Geometry check sheet. Reference: drawing and pictorial views, mm from the part's lowest x, y, z. A direction names the side the tool comes from. Round coordinates to 2 decimals unless told otherwise and drop trailing zeros. Order: outer loops, then holes, each group sorted by start corner. A loop starts at its lowest first (then second) coordinate and runs counter-clockwise, first axis right, second up. Notation, with made-up numbers: M -35.5,82 L 6.5,82 A21 cw 6.5,90 Z; hole C 45.25,28 d8. An arc over 180 degrees is marked long. Answer as a JSON object with one key per item and string values. Group by question number.
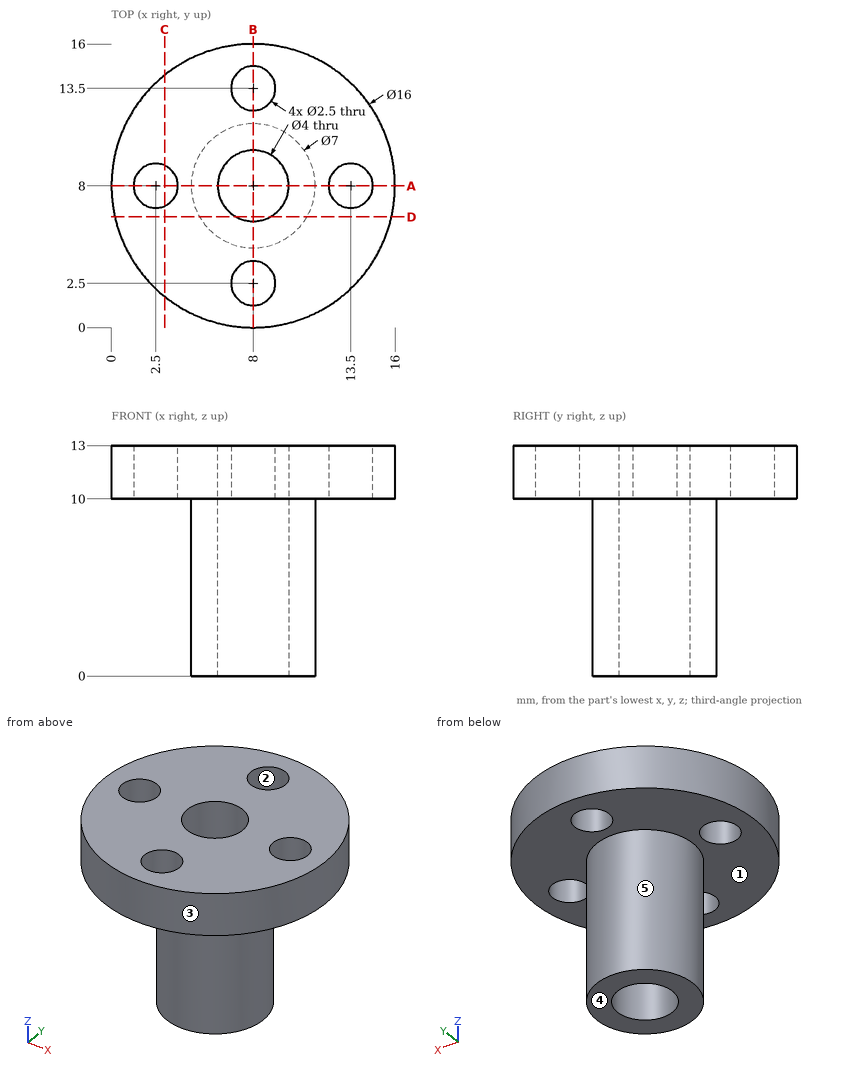
Q1. Tool access check on the marked faces 4 and 5. Record the directions out of +Z, -Z, +X, -X, +Y, -Y that give a thin tool (end or side, any length) a straight path to the whole face; none if there is none.
Q2. Gauge pin test, flat ends, axial feed: pin 1 Ø6 at (x, z) = (6.5, 11.5) entering from -Y; pin 2 Ø3 at (x, y) = (8, 2.5) entering from -Z; pin 3 Ø5 at (y, z) = (8, 1.5) entering from -X; pin 4 Ø4 at (y, z) = (11, 10.5) entering from -X. Record the tip position at first contact, or that the pin passes through.
Q3. Cross-section at D-D, the plane y = 6.25. Record the cut outline in (x, z).
Q4. Cross-section at C-C, the plane x = 3. Record the cut outline in (y, z) (3 decimals), then the cut area to 3 significant figures.
Q5. Release check for a two-part mould opening along X. For the marked faces 1, 2 and 3 record: released by +X, released by -X, zero draft, split by the parting line, or undercut.
Q6. Thickness scan on line 1 (Y direction, x = 8, z = 3.75); line 2 (Z direction, x = 6.5, y = 1.5); line 3 (Y direction, x = 3.5, z = 10.25). Record the ranges inside material, lowest first. Write a range as from..to.
Q7. Cross-section at A-A, the plane y = 8. Record the cut outline in (x, z), then the cut area to 3 significant figures.
Conclusion:
{
 "1": {"face 4": "-Z, +X, -X, +Y, -Y", "face 5": "-Z"},
 "2": {"pin 1": "y = 0", "pin 2": "z = 10", "pin 3": "x = 4.5", "pin 4": "x = 0.06"},
 "3": {"outline": "M 0.19,10 L 4.97,10 L 4.97,0 L 7.03,0 L 7.03,13 L 0.19,13 Z; M 8.97,0 L 11.03,0 L 11.03,10 L 15.81,10 L 15.81,13 L 8.97,13 Z"},
 "4": {"outline": "M 1.755,10 L 6.854,10 L 6.854,13 L 1.755,13 Z; M 9.146,10 L 14.245,10 L 14.245,13 L 9.146,13 Z", "area": "30.6 mm2"},
 "5": {"face 1": "zero draft", "face 2": "undercut", "face 3": "split by the parting line"},
 "6": {"line 1": "4.5..6, 10..11.5", "line 2": "10..13", "line 3": "1.39..7.25, 8.75..14.61"},
 "7": {"outline": "M 0,10 L 1.25,10 L 1.25,13 L 0,13 Z; M 3.75,10 L 4.5,10 L 4.5,0 L 6,0 L 6,13 L 3.75,13 Z; M 10,0 L 11.5,0 L 11.5,10 L 12.25,10 L 12.25,13 L 10,13 Z; M 14.75,10 L 16,10 L 16,13 L 14.75,13 Z", "area": "51.0 mm2"}
}
